from build123d import *

# Parameters (mm, degrees)
HEX_CUT_DEPTH = 3.175


with BuildPart() as part:
    # Sketch1 → Screw revolve (revolve)
    with BuildSketch(Plane.XY):
        with BuildLine():
            Line((0, 0), (3.175, 0))
            Line((3.175, 0), (3.175, 9.525))
            Line((3.175, 9.525), (6.858, 9.525))
            Line((6.858, 9.525), (6.858, 10.541))
            Line((6.858, 10.541), (5.334, 10.541))
            ThreePointArc((5.334, 10.541), (3.980323293, 11.907132143), (2.291358881, 12.827))
            Line((2.291358881, 12.827), (0, 12.827))
            Line((0, 12.827), (0, 0))
        make_face()
    revolve(axis=Axis((0, 0, 0), (0, 1, 0)))

    # Sketch2 → Hex Cut (cut)
    with BuildSketch(Plane(origin=(0, 12.827, 0), x_dir=(-1, 0, 0), z_dir=(0, 1, 0))):
        Polygon((-2.291358881, 0), (-1.14567944, -1.984375), (1.14567944, -1.984375), (2.291358881, 0), (1.14567944, 1.984375), (-1.14567944, 1.984375), align=None)
    extrude(amount=-HEX_CUT_DEPTH, mode=Mode.SUBTRACT)


solid = part.part
Geometry check sheet. Reference: the model listing, model coordinates, mm. A direction names the side the tool comes from. Round coordinates to 2 decimals unless told otherwise and drop trailing zeros. Write each loop counter-clockwise with the first axis right and the second up, starting at its lowest first coordinate (ties: lowest second). Pieces come first, ordered by that corner, then holes. Notation, with made-up numbers: (-9.5, 35) - (-5.5, 35) arc R30 ccw to (-5.5, 62) - close; hole circle Ø9 at (71.5, 0). An arc over 180 degrees is marked (long way). One line per item, written item: value.
1. Scan lines: L1, parallel to Y at x = 5, z = 2.75 (3 decimals); L2, parallel to Z at x = 1.25, y = 9.75; L3, parallel to Y at x = 1.5, z = 0. Record each from-to range of solid material in increasing order.
The answers:
L1: y = 9.525 to 10.541
L2: z = -6.74 to -1.8, 1.8 to 6.74
L3: y = 0 to 9.65
2. Cross-section at C-C on y = 11.75. Record the boundary of the cut face in (x, z).
The answers:
outline: circle Ø8.36 at (0, 0); hole (-2.29, 0) - (-1.15, -1.98) - (1.15, -1.98) - (2.29, 0) - (1.15, 1.98) - (-1.15, 1.98) - close
3. Depth check by flat-ended pin: pin 1 Ø2 at (x, z) = (-4, 4.5) entering from +Y; pin 2 Ø0.7 at (x, y) = (0, 11) entering from -Z; pin 3 Ø3 at (x, z) = (3.5, 5.5) entering from -Y (3 decimals). Enter the tip coordinate at first touch or a pass-through.
The answers:
pin 1: stops at y = 10.93
pin 2: stops at z = -5.25
pin 3: stops at y = 9.525
4. Cross-section at D-D on y = 8.75. Record the boundary of the cut face in (x, z) (3 decimals), and give its area (3 significant figures).
The answers:
outline: circle Ø6.35 at (0, 0)
area: 31.7 mm^2
5. Cross-section at A-A on x = 0. Record the boundary of the cut face in (y, z) (3 decimals).
The answers:
outline: (0, -3.175) - (9.525, -3.175) - (9.525, -6.858) - (10.541, -6.858) - (10.541, -5.334) arc R6.626 ccw to (12.827, -2.291) - (12.827, -1.984) - (9.652, -1.984) - (9.652, 1.984) - (12.827, 1.984) - (12.827, 2.291) arc R6.626 ccw to (10.541, 5.334) - (10.541, 6.858) - (9.525, 6.858) - (9.525, 3.175) - (0, 3.175) - close
6. Mould release check, pull along X, two halves, no side actions. Record for faces 1 (the face through (1.727, 11.262, -0.978)), 2 (the face through (-0.69, 4.83, 3.1)), 3 (the face through (4, 10.541, 4)): released by +X, released by -X, zero draft, split by the parting line, or undercut.
The answers:
face 1: undercut
face 2: split by the parting line
face 3: zero draft
7. Set-up check for faces 4 (the face through (-1.487, 10.04, 6.695)), 5 (the face through (0, 11, 1.984)), 6 (the face through (-3, 9.525, -2)): record each of +Z, -Z, +X, -X, +Y, -Y from which the full face is reachable in a straight line by a thin tool's end or side.
The answers:
face 4: +Y, -Y
face 5: +Y
face 6: -Y
8. Cross-section at B-B on z = 2.75. Record the boundary of the cut face in (x, y) (3 decimals).
The answers:
outline: (-6.282, 9.525) - (-1.587, 9.525) - (-1.587, 0) - (1.587, 0) - (1.587, 9.525) - (6.282, 9.525) - (6.282, 10.541) - (4.57, 10.541) arc R6.029 ccw to (-4.57, 10.541) - (-6.282, 10.541) - close
